Build history of the part. All positions in model axes, mm. Face numbers are marked on the shaded views. Coordinates: 2 decimals unless noted, no trailing zeros. Order: outer loops, then holes, each group sorted by start corner. A loop starts at its lowest first (then second) coordinate and runs counter-clockwise, first axis right, second up. Notation, with made-up numbers: (69.5, 21.25) - (113.5, 21.25) arc R13 cw to (113.5, 40.25) - close; hole circle Ø4 at (59.25, 45.25). An arc over 180 degrees is marked (long way). One line per item, written item: value.
from build123d import *

# Parameters (mm, degrees)
SKETCH1_W           = 12
SKETCH1_H           = 11
BOSS_EXTRUDE1_DEPTH = 1.6
SKETCH2_W           = 12
SKETCH2_H           = 11
BOSS_EXTRUDE2_DEPTH = 2
CUT_EXTRUDE1_DEPTH  = 17.672132437
CUT_EXTRUDE2_DEPTH  = 17.672132437
FILLET1_R           = 1


with BuildPart() as part:
    # Sketch1 → Boss-Extrude1 (new body)
    with BuildSketch(Plane(origin=(0, 0, 0), x_dir=(1, 0, 0), z_dir=(0, 1, 0))):
        with Locations((6, -5.5)):
            Rectangle(SKETCH1_W, SKETCH1_H)
    extrude(amount=BOSS_EXTRUDE1_DEPTH)

    # Sketch2 → Boss-Extrude2 (add)
    with BuildSketch(Plane(origin=(0, 1.6, 0), x_dir=(1, 0, 0), z_dir=(0, 1, 0))):
        with Locations((6, -5.5)):
            Rectangle(SKETCH2_W, SKETCH2_H)
    extrude(amount=BOSS_EXTRUDE2_DEPTH)

    # Sketch3 → Cut-Extrude1 (cut, through all)
    with BuildSketch(Plane(origin=(12, 0, 0), x_dir=(0, 0, -1), z_dir=(1, 0, 0))):
        Polygon((-9.7, 1.9), (-8.2, 3.6), (-2.8, 3.6), (-1.3, 1.9), align=None)
    extrude(amount=-CUT_EXTRUDE1_DEPTH, mode=Mode.SUBTRACT)

    # Sketch4 → Cut-Extrude2 (cut, through all)
    with BuildSketch(Plane(origin=(12, 0, 0), x_dir=(0, 0, -1), z_dir=(1, 0, 0))):
        Polygon((-8.376470588, 3.4), (-8.376470588, 3.6), (-8.2, 3.6), align=None)
        Polygon((-2.623529412, 3.4), (-2.623529412, 3.6), (-2.8, 3.6), align=None)
    extrude(amount=-CUT_EXTRUDE2_DEPTH, mode=Mode.SUBTRACT)

    # Fillet1
    fillet1_edges = [part.edges().sort_by_distance(p)[0] for p in [
        (6, 3.6, 11),
        (6, 3.6, 0),
    ]]
    fillet(fillet1_edges, radius=FILLET1_R)


solid = part.part
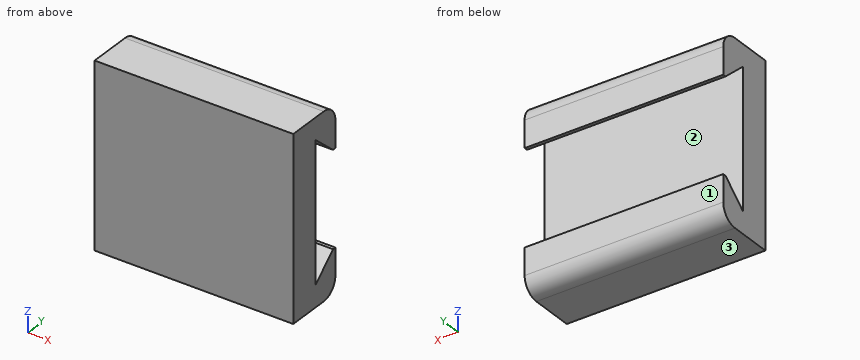
1. Band-saw the part on B-B, the plane x = 1. Give the cut face in (y, z), and give its area (3 significant figures).
Values found:
outline: (0, 0) - (2.6, 0) arc R1 ccw to (3.6, 1) - (3.6, 2.62) - (3.4, 2.62) - (1.9, 1.3) - (1.9, 9.7) - (3.4, 8.38) - (3.6, 8.38) - (3.6, 10) arc R1 ccw to (2.6, 11) - (0, 11) - close
area: 27.4 mm2
2. Band-saw the part on D-D, the plane z = 4.5. Give the cut face in (x, y), and give its area (3 significant figures).
Values found:
outline: (0, 0) - (12, 0) - (12, 1.9) - (0, 1.9) - close
area: 22.8 mm2
3. Band-saw the part on A-A, the plane z = 1.75. Give the cut face in (x, y).
Values found:
outline: (0, 0) - (12, 0) - (12, 1.9) - (0, 1.9) - close; (0, 2.41) - (12, 2.41) - (12, 3.6) - (0, 3.6) - close
4. Two-plate mould, pull along Y, no slides. Class the marked faces 1, 2 and 3: pulls with the +Y half, pulls with the -Y half, needs draft (parallel to the pull), parting line crosses it, or undercut.
Values found:
face 1: pulls with the +Y half
face 2: undercut
face 3: needs draft
5. Flat gauge pin, fed straight in: P1, Ø6, axis at x = 6, z = 3.5, coming from the -Y side. Where does the tip first touch, or does it go through?
Values found:
P1: stops at y = 0
6. Probe line 1 along Y through (x, z) = (8.75, 4); line 2 along Z through (x, y) = (11, 3.3); line 3 along Y through (x, z) = (11.5, 9.25). List the from-to ranges inside material, lowest first.
Values found:
line 1: y = 0 to 1.9
line 2: z = 0.29 to 2.54, 8.46 to 10.71
line 3: y = 0 to 1.9, 2.41 to 3.6
7. Band-saw the part on C-C, the plane y = 2.75. Give the cut face in (x, z).
Values found:
outline: (0, 0.01) - (12, 0.01) - (12, 2.05) - (0, 2.05) - close; (0, 8.95) - (12, 8.95) - (12, 10.99) - (0, 10.99) - close
